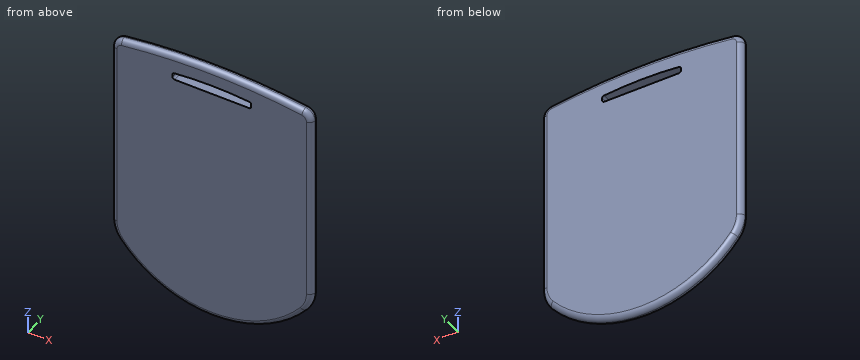
from build123d import *

# Parameters (mm, degrees)
BOSS_EXTRUDE1_DEPTH = 10
FILLET1_R           = 5


with BuildPart() as part:
    # Sketch1 → Boss-Extrude1 (new body)
    with BuildSketch(Plane(origin=(0, 0, 0), x_dir=(1, 0, 0), z_dir=(0, 1, 0))):
        with BuildLine():
            Line((95.064475679, -66.893222563), (95.064480767, 108.106777437))
            ThreePointArc((95.064480767, 108.106777437), (93.254744528, 118.406620299), (88.04232554, 127.472633565))
            ThreePointArc((88.04232554, 127.472633565), (-0.544574451, 168.543910176), (-88.562996968, 126.268078898))
            ThreePointArc((-88.562996968, 126.268078898), (-93.583004489, 117.32624486), (-95.323148669, 107.220366882))
            Line((-95.323148669, 107.220366882), (-95.323030776, -67.779633118))
            ThreePointArc((-95.323030776, -67.779633118), (-92.800151785, -74.512215926), (-86.474089698, -77.92887045))
            ThreePointArc((-86.474089698, -77.92887045), (-0.044332377, -83.617951425), (86.321358486, -77.027349436))
            ThreePointArc((86.321358486, -77.027349436), (92.576619033, -73.585431127), (95.064475679, -66.893222563))
        make_face()
        with BuildLine():
            Line((35.5, -58.821440939), (-35.5, -58.821440939))
            ThreePointArc((-35.5, -58.821440939), (-36.914213562, -59.407227376), (-37.5, -60.821440939))
            Line((-37.5, -60.821440939), (-37.5, -63.222008463))
            ThreePointArc((-37.5, -63.222008463), (-36.98495569, -64.561749706), (-35.705093402, -65.211464845))
            ThreePointArc((-35.705093402, -65.211464845), (0, -67.047022968), (35.705093402, -65.211464845))
            ThreePointArc((35.705093402, -65.211464845), (36.98495569, -64.561749706), (37.5, -63.222008463))
            Line((37.5, -63.222008463), (37.5, -60.821440939))
            ThreePointArc((37.5, -60.821440939), (36.914213562, -59.407227376), (35.5, -58.821440939))
        make_face(mode=Mode.SUBTRACT)
    extrude(amount=BOSS_EXTRUDE1_DEPTH)

    # Fillet1
    fillet1_edges = [part.edges().sort_by_distance(p)[0] for p in [
        (92.576619033, 10, 73.585431127),
        (-0.044332377, 10, 83.617951425),
        (-92.800151785, 10, 74.512215926),
        (-95.323089722, 10, -19.720366882),
        (-93.583004489, 10, -117.32624486),
        (-0.544574451, 10, -168.543910176),
        (93.254744528, 10, -118.406620299),
        (92.576619033, 0, 73.585431127),
        (-0.044332377, 0, 83.617951425),
        (-92.800151785, 0, 74.512215926),
        (-95.323089722, 0, -19.720366882),
        (-93.583004489, 0, -117.32624486),
        (-0.544574451, 0, -168.543910176),
        (93.254744528, 0, -118.406620299),
        (95.064478223, 10, -20.606777437),
        (95.064478223, 0, -20.606777437),
    ]]
    fillet(fillet1_edges, radius=FILLET1_R - 0.0001)  # a hair under: the kernel refuses the full size


solid = part.part
Could you check a few things on this model? Use its own coordinates, in mm. Give positions to 0.01 mm unless a question says otherwise; leave off trailing zeros. Order: outer loops, then holes, each group sorted by start corner. A loop starts at its lowest first (then second) coordinate and runs counter-clockwise, first axis right, second up. Notation, with made-up numbers: M -26,62 L 7,62 A15 cw 7,67 Z; hole C 77.5,35 d4. An arc over 180 degrees is marked long. One line per question, with ' | ' between items.
1. If I drill on line 1 (X direction, y = 4.5, z = 60.5); line 2 (Z direction, x = -14.5, y = 7.75); line 3 (Z direction, x = -24, y = 3.75), over which ranges is the centre line in solid material (lowest first)?
Results:
line 1: -95.3 to -37.47, 37.47 to 95.04 | line 2: -166.76 to 58.82, 66.74 to 82.7 | line 3: -165.79 to 58.82, 66.22 to 83.11
2. I want a section at A-A (y = 3.25). List the corners of the cut face in (x, z) for me (3 decimals).
Results:
outline: M -95.007,-107.22 A29.899 ccw -88.318,-126.069 A114.076 ccw 87.8,-127.27 A29.899 ccw 94.748,-108.107 L 94.748,66.893 A9.929 ccw 86.275,76.715 A610.641 ccw -86.431,77.616 A9.929 ccw -95.007,67.78 Z; hole M -37.5,60.821 A2 ccw -35.5,58.821 L 35.5,58.821 A2 ccw 37.5,60.821 L 37.5,63.222 A2 ccw 35.705,65.211 A348.184 ccw -35.705,65.211 A2 ccw -37.5,63.222 Z
3. I'm going to push flat-ended pins straight in: pin 1 (1.5 mm diameter, centred on y = 1.5, z = -10, fed in from -X); pin 2 (5 mm diameter, centred on x = -54.5, z = -24.5, fed in from -Y); pin 3 (1.5 mm diameter, centred on y = 2, z = -68.5, fed in from +X); pin 4 (1 mm diameter, centred on y = 8, z = -122.5, fed in from +X). Where does each tip first touch, or does it pass through?
Results:
pin 1: x = -94.5 | pin 2: y = 0 | pin 3: x = 94.53 | pin 4: x = 90.75
